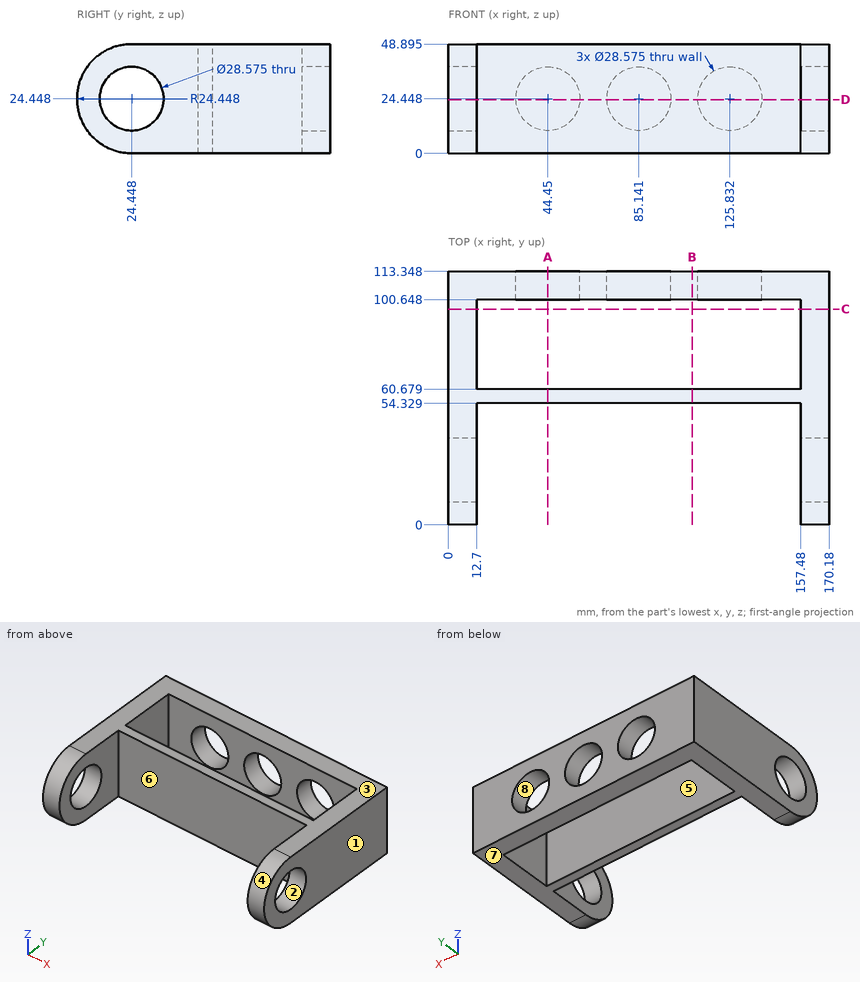
Input: dimensioned drawing with shaded views. Units: mm. Origin: part minimum x, y, z. A direction names the side the tool comes from. Coordinates: 2 decimals unless noted, no trailing zeros. Write each loop counter-clockwise with the first axis right and the second up, starting at its lowest first coordinate (ties: lowest second). Pieces come first, ordered by that corner, then holes. Notation, with made-up numbers: M 70,29.5 L 114,29.5 A18 cw 114,41.5 Z; hole C 35,67 d3. An arc over 180 degrees is marked long. Use a Markdown table: item, result.
1) Section A-A, the plane x = 44.45. Output: boundary loops of the cut face in (y, z) (1 decimal).
Conclusion:
| item | result |
|---|---|
| outline | M 54.3,0 L 60.7,0 L 60.7,48.9 L 54.3,48.9 Z; M 100.6,0 L 113.3,0 L 113.3,10.2 L 100.6,10.2 Z; M 100.6,38.7 L 113.3,38.7 L 113.3,48.9 L 100.6,48.9 Z |
2) Section B-B, the plane x = 109. Output: boundary loops of the cut face in (y, z) (1 decimal).
Conclusion:
| item | result |
|---|---|
| outline | M 54.3,0 L 60.7,0 L 60.7,48.9 L 54.3,48.9 Z; M 100.6,0 L 113.3,0 L 113.3,48.9 L 100.6,48.9 Z |
3) Section D-D, the plane z = 24. Give the number of separate pieces and of enclosed holes in the cut face, then the cut area to 3 significant figures.
Conclusion:
| item | result |
|---|---|
| separate pieces | 5 |
| enclosed holes | 0 |
| area | 3,820 mm^2 |
4) First-contact query: pin 1 Ø23 at (x, z) = (85.14, 24.45) entering from -Y; pin 2 Ø1.5 at (x, z) = (46, 30) entering from +Y. Flat tips, straight axial feed; report the tip coordinate or a pass-through.
Conclusion:
| item | result |
|---|---|
| pin 1 | stops at y = 54.33 |
| pin 2 | stops at y = 60.68 |
5) Section C-C, the plane y = 96.5. Output: boundary loops of the cut face in (x, z) (1 decimal), then the cut area to 3 significant figures.
Conclusion:
| item | result |
|---|---|
| outline | M 0,0 L 12.7,0 L 12.7,48.9 L 0,48.9 Z; M 157.5,0 L 170.2,0 L 170.2,48.9 L 157.5,48.9 Z |
| area | 1,240 mm^2 |
6) Ray query, L1, parallel to Y at x = 143, z = 23; L2, parallel to X at y = 88, z = 35; L3, parallel to Y at x = 134.5, z = 27. Return the intervals inside material, ascending.
Conclusion:
| item | result |
|---|---|
| L1 | y = 54.33 to 60.68, 100.65 to 113.35 |
| L2 | x = 0 to 12.7, 157.48 to 170.18 |
| L3 | y = 54.33 to 60.68 |
7) Reachability of the marked faces 4, 5, 6, 7 and 8 from +Z, -Z, +X, -X, +Y, -Y: full face, straight path, thin tool, end or side. Return the list, or none.
Conclusion:
| item | result |
|---|---|
| face 4 | +X, -X, -Y |
| face 5 | +Z, -Z |
| face 6 | +Z, -Z, -Y |
| face 7 | -Z, +X, -X, +Y, -Y |
| face 8 | +Y |
8) Mould query, pull axis Z, two halves, no side actions, for the marked faces 1, 2 and 3. Classes: pulls with the +Z half, pulls with the -Z half, needs draft (parallel to the pull), parting line crosses it, or undercut.
Conclusion:
| item | result |
|---|---|
| face 1 | needs draft |
| face 2 | undercut |
| face 3 | pulls with the +Z half |
